The listing builds one solid part. Answer for the finished solid, in the listing's coordinates (mm). A direction names the side the tool comes from. Give positions to 0.01 mm unless a question says otherwise; leave off trailing zeros. Write each loop counter-clockwise with the first axis right and the second up, starting at its lowest first coordinate (ties: lowest second). Pieces come first, ordered by that corner, then holes. Notation, with made-up numbers: (19.5, 79.25) - (37.5, 79.25) arc R26 ccw to (37.5, 98.25) - close; hole circle Ø9 at (33, 27.5). An arc over 180 degrees is marked (long way). Answer in a Markdown table with one row per item. Add a question column.
from build123d import *

# Parameters (mm, degrees)
SKETCH1_W           = 60
SKETCH1_H           = 50
SKETCH1_R           = 12.5
BOSS_EXTRUDE1_DEPTH = 4
CUT_EXTRUDE1_DEPTH  = 5


with BuildPart() as part:
    # Sketch1 → Boss-Extrude1 (new body)
    with BuildSketch(Plane.XY):
        Rectangle(SKETCH1_W, SKETCH1_H)
        Circle(SKETCH1_R, mode=Mode.SUBTRACT)
    extrude(amount=BOSS_EXTRUDE1_DEPTH)

    # Sketch2 → Cut-Extrude1 (cut, through all)
    with BuildSketch(Plane.XY.offset(4)):
        Polygon((-17.5, -5), (-22.5, -5), (-22.5, -10.5), (-25, -10.5), (-25, -15.5), (-22.5, -15.5), (-22.5, -25), (-17.5, -25), (-17.5, -15.5), (-15, -15.5), (-15, -10.5), (-17.5, -10.5), align=None)
        Polygon((22.5, -5), (17.5, -5), (17.5, -10.5), (15, -10.5), (15, -15.5), (17.5, -15.5), (17.5, -25), (22.5, -25), (22.5, -15.5), (25, -15.5), (25, -10.5), (22.5, -10.5), align=None)
    extrude(amount=-CUT_EXTRUDE1_DEPTH, mode=Mode.SUBTRACT)


solid = part.part
1. The mould has two halves that part along X. Classify faces 4 (the face through (30, 0, 2)), 5 (the face through (-17.5, -20, 2)), 6 (the face through (0, 25, 2)): +X half, -X half, draft (parallel to the pull), parting line (faces both ways), or undercut.
2. A tool of negligible diameter and unlimited length cuts with its end or side. For faces 1 (the face through (-7, 11, 4)), 2 (the face through (-22.5, -20, 2)), 3 (the face through (24, -10.5, 2)), from which of +Z, -Z, +X, -X, +Y, -Y can it reach the whole face along a straight path? Write none if from no direction.
3. Section B-B (y = -17.5) is taken. Give the vertices of the cut face in (x, z).
4. Straight lines are drawn through the part: L1, parallel to X at y = -14.5, z = 1.55; L2, parallel to Y at x = 0, z = 2.95; L3, parallel to X at y = 0.5, z = 3.15. For each, find the intervals that lie inside material, in ascending order. Write a range as [from, to].
5. Given pin 1 Ø1.2 at (x, z) = (19, 1.5) entering from -Y, flat-ended and moving along its own axis, determine where the tip first touches the part or whether it passes through.
6. Section A-A (x = -24) is taken. Give the vertices of the cut face in (y, z).
7. Section D-D (y = 0) is taken. Give the vertices of the cut face in (x, z).
Geometry check:
| question | item | result |
|---|---|---|
| 1 | face 4 | +X half |
| 1 | face 5 | undercut |
| 1 | face 6 | draft |
| 2 | face 1 | +Z, +X, -X, +Y, -Y |
| 2 | face 2 | +Z, -Z, -Y |
| 2 | face 3 | +Z, -Z |
| 3 | outline | (-30, 0) - (-22.5, 0) - (-22.5, 4) - (-30, 4) - close; (-17.5, 0) - (17.5, 0) - (17.5, 4) - (-17.5, 4) - close; (22.5, 0) - (30, 0) - (30, 4) - (22.5, 4) - close |
| 4 | L1 | [-30, -25], [-15, 15], [25, 30] |
| 4 | L2 | [-25, -12.5], [12.5, 25] |
| 4 | L3 | [-30, -12.49], [12.49, 30] |
| 5 | pin 1 | y = -5 |
| 6 | outline | (-25, 0) - (-15.5, 0) - (-15.5, 4) - (-25, 4) - close; (-10.5, 0) - (25, 0) - (25, 4) - (-10.5, 4) - close |
| 7 | outline | (-30, 0) - (-12.5, 0) - (-12.5, 4) - (-30, 4) - close; (12.5, 0) - (30, 0) - (30, 4) - (12.5, 4) - close |
